```python
from build123d import *

# Parameters (mm, degrees)
SKETCH_1_R      = 0.75
EXTRUDE_1_DEPTH = 1.1


with BuildPart() as part:
    # 草图1 → 凸台-拉伸1 (new body)
    with BuildSketch(Plane.XY):
        with BuildLine():
            Line((-1, -9.142997198), (-1, -5.808326913))
            ThreePointArc((-1, -5.808326913), (-3.51781182, 3.827883631), (5.5, -0.4))
            ThreePointArc((5.5, -0.4), (4.227883631, -3.91781182), (1, -5.808326913))
            Line((1, -5.808326913), (1, -9.142997198))
            ThreePointArc((1, -9.142997198), (2.711468806, -8.771853852), (4.315554735, -8.069158189))
            ThreePointArc((4.315554735, -8.069158189), (4.380668311, -8.010477473), (4.414435496, -7.929588775))
            Line((4.414435496, -7.929588775), (4.975043576, -4.75022236))
            ThreePointArc((4.975043576, -4.75022236), (5.017096746, -4.619827111), (5.092964751, -4.505741898))
            ThreePointArc((5.092964751, -4.505741898), (0, 6.8), (-5.092964751, -4.505741898))
            ThreePointArc((-5.092964751, -4.505741898), (-5.017096746, -4.619827111), (-4.975043576, -4.75022236))
            Line((-4.975043576, -4.75022236), (-4.414435496, -7.929588775))
            ThreePointArc((-4.414435496, -7.929588775), (-4.380668311, -8.010477473), (-4.315554735, -8.069158189))
            ThreePointArc((-4.315554735, -8.069158189), (-2.711468806, -8.771853852), (-1, -9.142997198))
        make_face()
        with Locations((-3, -7.093477568)):
            Circle(SKETCH_1_R, mode=Mode.SUBTRACT)
        with Locations((3, -7.093477568)):
            Circle(SKETCH_1_R, mode=Mode.SUBTRACT)
    extrude(amount=EXTRUDE_1_DEPTH)


solid = part.part
```
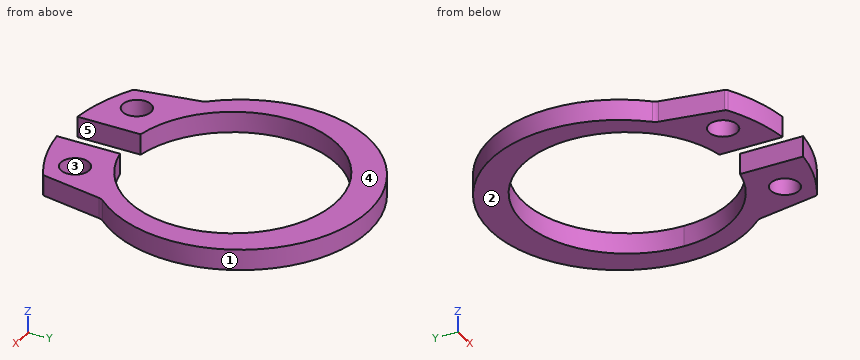
The model under review builds one solid part; all positions refer to its coordinate system, in mm. Face numbers are marked on the shaded views. A direction names the side the tool comes from. Round coordinates to 2 decimals unless told otherwise and drop trailing zeros. Write each loop counter-clockwise with the first axis right and the second up, starting at its lowest first coordinate (ties: lowest second). Pieces come first, ordered by that corner, then holes. Notation, with made-up numbers: (-9.75, -3) - (17.25, -3) arc R18 cw to (17.25, 29) - close; hole circle Ø7 at (89.5, 33). An arc over 180 degrees is marked (long way). Answer as CSV lines item,"result". Start each with the question number.
(1) To check wall thickness, follow line 1 (X direction, y = -6.5, z = 1); line 2 (Y direction, x = 3, z = 0.7); line 3 (X direction, y = -0.25, z = 0.8). State the ranges of each line that lie inside material, in increasing order.
(2) We need section C-C on x = -1.5. State the section outline as (y, z) points, plus the area to 3 significant figures.
(3) We need section B-B on z = 0.2. State the section outline as (x, y) points.
(4) Draft analysis for pull direction X (two halves, no side actions). For the marked faces 1, 2 and 3, state which applies: pulls with the +X half, pulls with the -X half, needs draft (parallel to the pull), parting line crosses it, or undercut.
(5) For pin 1 Ø1.2 at (x, y) = (-3, -7.09) entering from +Z; pin 2 Ø0.6 at (y, z) = (-8, 0.5) entering from -X, all flat-tipped, find the tip position at first contact; note any pin that passes through.
(6) For the marked faces 4 and 5, list the 3-axis set-ups (+Z, -Z, +X, -X, +Y, -Y) from which the entire face can be reached by the end or side of a thin tool; tool diameter is ignored.
(7) We need section A-A on y = 0. State the section outline as (x, z) points.
(8) We need section D-D on x = 3. State the section outline as (y, z) points.
Worked answers:
1,line 1,"-4.67 to -3.46, -2.54 to -1, 1 to 2.54, 3.46 to 4.67"
1,line 2,"-8.67 to -7.84, -6.34 to -5.01, 4.21 to 6.1"
1,line 3,"-6.8 to -5.5, 5.5 to 6.8"
2,outline,"(-9.07, 0) - (-5.69, 0) - (-5.69, 1.1) - (-9.07, 1.1) - close; (4.89, 0) - (6.63, 0) - (6.63, 1.1) - (4.89, 1.1) - close"
2,area,"5.63 mm²"
3,outline,"(-5.09, -4.51) arc R0.5 cw to (-4.98, -4.75) - (-4.41, -7.93) arc R0.2 ccw to (-4.32, -8.07) arc R8.8 ccw to (-1, -9.14) - (-1, -5.81) arc R5.5 cw (long way) to (1, -5.81) - (1, -9.14) arc R8.8 ccw to (4.32, -8.07) arc R0.2 ccw to (4.41, -7.93) - (4.98, -4.75) arc R0.5 cw to (5.09, -4.51) arc R6.8 ccw (long way) to start; hole circle Ø1.5 at (-3, -7.09); hole circle Ø1.5 at (3, -7.09)"
4,face 1,"parting line crosses it"
4,face 2,"needs draft"
4,face 3,"undercut"
5,pin 1,"through"
5,pin 2,"x = -4.45"
6,face 4,"+Z, +X, -X, +Y, -Y"
6,face 5,"+Z, -Z, -Y"
7,outline,"(-6.8, 0) - (-5.49, 0) - (-5.49, 1.1) - (-6.8, 1.1) - close; (5.49, 0) - (6.8, 0) - (6.8, 1.1) - (5.49, 1.1) - close"
8,outline,"(-8.67, 0) - (-7.84, 0) - (-7.84, 1.1) - (-8.67, 1.1) - close; (-6.34, 0) - (-5.01, 0) - (-5.01, 1.1) - (-6.34, 1.1) - close; (4.21, 0) - (6.1, 0) - (6.1, 1.1) - (4.21, 1.1) - close"
